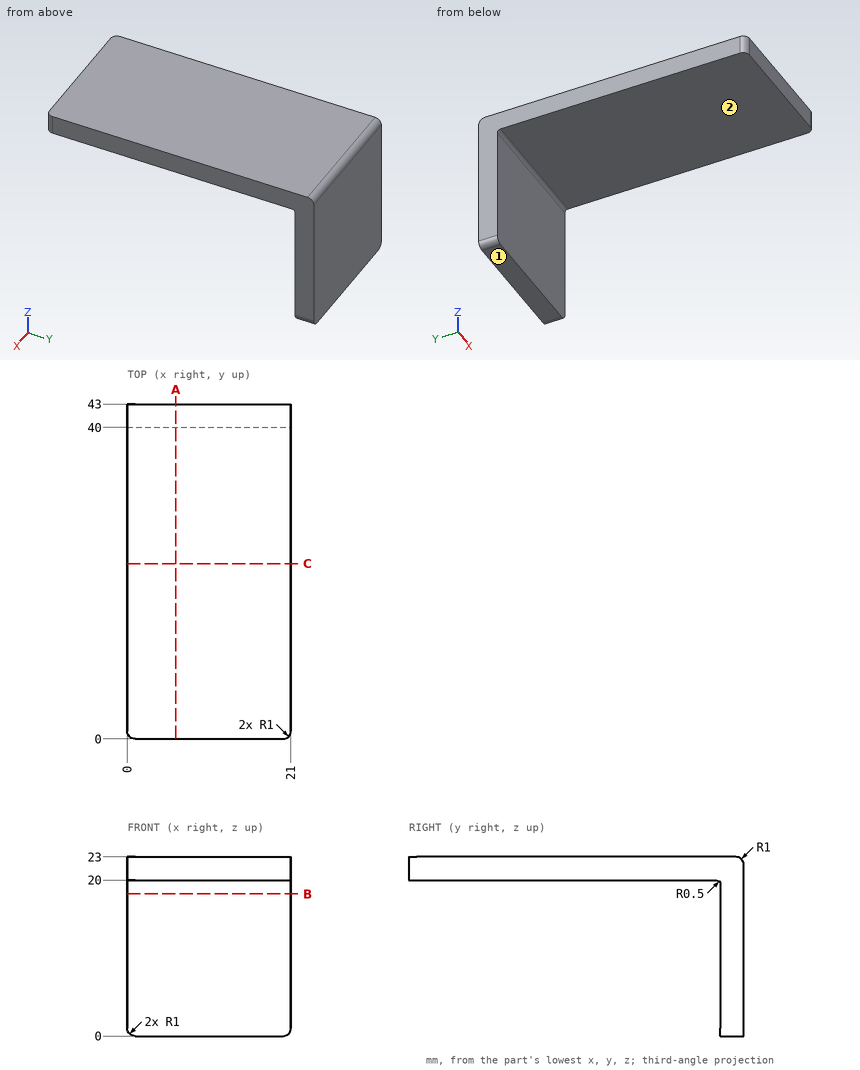
Job drawing, mm, ordinate dimensions from the low corner. One solid piece. A direction names the side the tool comes from. Give positions to 0.01 mm unless a question says otherwise; leave off trailing zeros. Loops run counter-clockwise (first coordinate to the right, second up) from the corner with the lowest first, then second, coordinate; pieces in that order, holes last. Notation, with made-up numbers: (42.5, 76) - (97.5, 76) arc R28 ccw to (97.5, 102) - close; hole circle Ø6 at (27.5, 14). An arc over 180 degrees is marked (long way). Use one line per item in the form item = value.
(1) Cut at C-C (y = 22.5). Give the cut face in (x, z), then the cut area to 3 significant figures.
Determined:
outline = (0, 20) - (21, 20) - (21, 23) - (0, 23) - close
area = 63.0 mm^2
(2) Cut at A-A (x = 6.25). Give the cut face in (y, z), then the cut area to 3 significant figures.
Determined:
outline = (0, 20) - (39.5, 20) arc R0.5 cw to (40, 19.5) - (40, 0) - (43, 0) - (43, 22) arc R1 ccw to (42, 23) - (0, 23) - close
area = 189 mm^2
(3) 3-axis set-ups, long thin cutter, end or side, ignore diameter. For the marked faces 1 and 2: which of +Z, -Z, +X, -X, +Y, -Y reach the whole face in a straight line?
Determined:
face_1 = -Z, +X, -X, +Y, -Y
face_2 = -Z, +X, -X, -Y
(4) Drop a flat-ended pin along its axis: P1, Ø6, axis at x = 12.5, y = 31.5, coming from the -Z side. Give the stop position or say it passes through.
Determined:
P1 = 20
(5) Cut at B-B (z = 18.25). Give the cut face in (x, y).
Determined:
outline = (0, 40) - (21, 40) - (21, 43) - (0, 43) - close
(6) Drill centre lines: L1, parallel to Y at x = 3, z = 16; L2, parallel to Z at x = 19.5, y = 13.5. Where is each one in solid material? Low to high.
Determined:
L1 = 40 to 43
L2 = 20 to 23
